from build123d import *

# Parameters (mm, degrees)
SKETCH2_R          = 17
EXTRUSION4_DEPTH   = 10
SKETCH3_R          = 9.15
EXTRUSION5_DEPTH   = 5
FILLET2_R          = 1
FILLET3_R          = 2
FILLET4_R          = 1
FILLET5_R          = 1
SKETCH4_R          = 2.75
CUT_EXTRUDE3_DEPTH = 12
SKETCH5_R          = 3.25
CUT_EXTRUDE4_DEPTH = 1


with BuildPart() as part:
    # Sketch1 → Revolution1 (revolve)
    with BuildSketch(Plane.XY, mode=Mode.PRIVATE) as revolution1_sk:
        Polygon((17, 0), (17, 106), (20, 106), (20, 110), (0, 110), (0, 0), align=None)
    revolve(revolution1_sk.sketch.rotate(Axis((0, 0, 0), (0, 1, 0)), 90), axis=Axis((0, 0, 0), (0, 1, 0)))

    # Sketch2 → Extrusion4 (add)
    with BuildSketch(Plane.XZ):
        with Locations(Location((0, 0, 0), (0, 0, 270))):
            Circle(SKETCH2_R)
    extrude(amount=EXTRUSION4_DEPTH)

    # Sketch3 → Extrusion5 (cut)
    with BuildSketch(Plane(origin=(0, 110, 0), x_dir=(-1, 0, 0), z_dir=(0, 1, 0))):
        with Locations(Location((0, 0, 0), (0, 0, 90))):
            Circle(SKETCH3_R)
    extrude(amount=-EXTRUSION5_DEPTH, mode=Mode.SUBTRACT)

    # Fillet2
    fillet2_edges = [part.edges().sort_by_distance(p)[0] for p in [
        (0, 110, -9.15),
    ]]
    fillet(fillet2_edges, radius=FILLET2_R)

    # Fillet3
    fillet3_edges = [part.edges().sort_by_distance(p)[0] for p in [
        (0, 110, 20),
    ]]
    fillet(fillet3_edges, radius=FILLET3_R)

    # Fillet4
    fillet4_edges = [part.edges().sort_by_distance(p)[0] for p in [
        (0, 106, 20),
    ]]
    fillet(fillet4_edges, radius=FILLET4_R)

    # Fillet5
    fillet5_edges = [part.edges().sort_by_distance(p)[0] for p in [
        (0, 106, 17),
    ]]
    fillet(fillet5_edges, radius=FILLET5_R)

    # Sketch4 → Cut-Extrude3 (cut)
    with BuildSketch(Plane.XZ.offset(10)):
        with Locations(Location((0, 0, 0), (0, 0, 270))):
            Circle(SKETCH4_R)
    extrude(amount=-CUT_EXTRUDE3_DEPTH, mode=Mode.SUBTRACT)

    # Sketch5 → Cut-Extrude4 (cut)
    with BuildSketch(Plane.XZ.offset(10)):
        with Locations(Location((0, 0, 0), (0, 0, 270))):
            Circle(SKETCH5_R)
    extrude(amount=-CUT_EXTRUDE4_DEPTH, mode=Mode.SUBTRACT)


solid = part.part
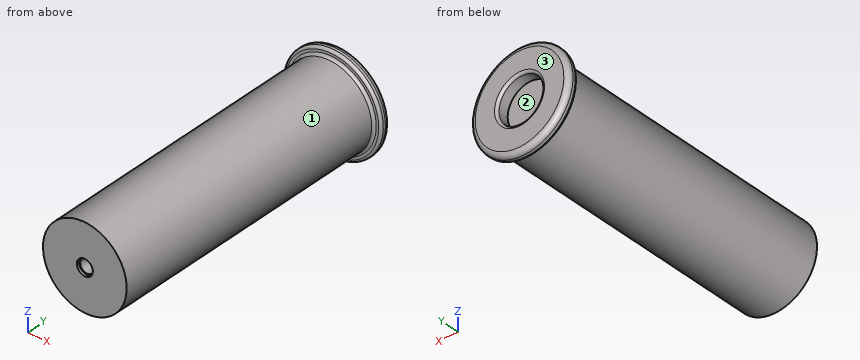
Input: part model. Units: mm. Frame: model coordinates. Face numbers are marked on the shaded views. Give positions to 0.01 mm unless a question says otherwise; leave off trailing zeros. Order: outer loops, then holes, each group sorted by start corner. A loop starts at its lowest first (then second) coordinate and runs counter-clockwise, first axis right, second up. Notation, with made-up numbers: (-27.5, -28) -> (2.5, -28) arc R13 cw to (2.5, -9) -> close; hole circle Ø1 at (43.25, 52). An arc over 180 degrees is marked (long way). Use one line per item in the form item = value.
1) First-contact query: pin 1 Ø9 at (x, z) = (0.5, 3.5) entering from +Y; pin 2 Ø1 at (x, y) = (6, 59) entering from +Z; pin 3 Ø24 at (x, z) = (0, 0) entering from -Y; pin 4 Ø2 at (y, z) = (17.5, -0.5) entering from -X. Flat tips, straight axial feed; report the tip coordinate or a pass-through.
Response values:
pin_1 = 105
pin_2 = 16.09
pin_3 = -10
pin_4 = -17
2) Section B-B, the plane y = -1.5. Return loops of the section in (x, z), and give its area (3 significant figures).
Response values:
outline = circle Ø34 at (0, 0); hole circle Ø5.5 at (0, 0)
area = 884 mm^2
3) Mould query, pull axis X, two halves, no side actions, for the marked faces 1, 2 and 3. Classes: pulls with the +X half, pulls with the -X half, needs draft (parallel to the pull), parting line crosses it, or undercut.
Response values:
face_1 = parting line crosses it
face_2 = undercut
face_3 = needs draft
4) Line query: probe 1 along X at (y, z) = (-4, 0); probe 2 along X at (y, z) = (-2, 1); probe 3 along Y at (x, z) = (17, 8). Output: solid intervals per line, ascending.
Response values:
probe_1 = -17 to -2.75, 2.75 to 17
probe_2 = -16.97 to -2.56, 2.56 to 16.97
probe_3 = 106 to 109.84
5) Section A-A, the plane x = 0. Return loops of the section in (y, z), and give its area (3 significant figures).
Response values:
outline = (-10, -17) -> (105, -17) arc R1 cw to (106, -18) -> (106, -19) arc R1 ccw to (107, -20) -> (108, -20) arc R2 ccw to (110, -18) -> (110, -10.15) arc R1 ccw to (109, -9.15) -> (105, -9.15) -> (105, 9.15) -> (109, 9.15) arc R1 ccw to (110, 10.15) -> (110, 18) arc R2 ccw to (108, 20) -> (107, 20) arc R1 ccw to (106, 19) -> (106, 18) arc R1 cw to (105, 17) -> (-10, 17) -> (-10, 3.25) -> (-9, 3.25) -> (-9, 2.75) -> (2, 2.75) -> (2, -2.75) -> (-9, -2.75) -> (-9, -3.25) -> (-10, -3.25) -> close
area = 3,940 mm^2
6) Section C-C, the plane z = 0. Return loops of the section in (x, y), and give its area (3 significant figures).
Response values:
outline = (-20, 107) arc R1 ccw to (-19, 106) -> (-18, 106) arc R1 cw to (-17, 105) -> (-17, -10) -> (-3.25, -10) -> (-3.25, -9) -> (-2.75, -9) -> (-2.75, 2) -> (2.75, 2) -> (2.75, -9) -> (3.25, -9) -> (3.25, -10) -> (17, -10) -> (17, 105) arc R1 cw to (18, 106) -> (19, 106) arc R1 ccw to (20, 107) -> (20, 108) arc R2 ccw to (18, 110) -> (10.15, 110) arc R1 ccw to (9.15, 109) -> (9.15, 105) -> (-9.15, 105) -> (-9.15, 109) arc R1 ccw to (-10.15, 110) -> (-18, 110) arc R2 ccw to (-20, 108) -> close
area = 3,940 mm^2
7) Section D-D, the plane y = 101.5. Return loops of the section in (x, z).
Response values:
outline = circle Ø34 at (0, 0)
